Geometry check sheet. Reference: drawing and pictorial views, mm from the part's lowest x, y, z. A direction names the side the tool comes from. Round coordinates to 2 decimals unless told otherwise and drop trailing zeros. Write each loop counter-clockwise with the first axis right and the second up, starting at its lowest first coordinate (ties: lowest second). Pieces come first, ordered by that corner, then holes. Notation, with made-up numbers: (67.5, 11) - (101.5, 11) arc R21 ccw to (101.5, 38) - close; hole circle Ø10 at (6.25, -18.75). An arc over 180 degrees is marked (long way). Return JSON: item names as keys, results as strings.
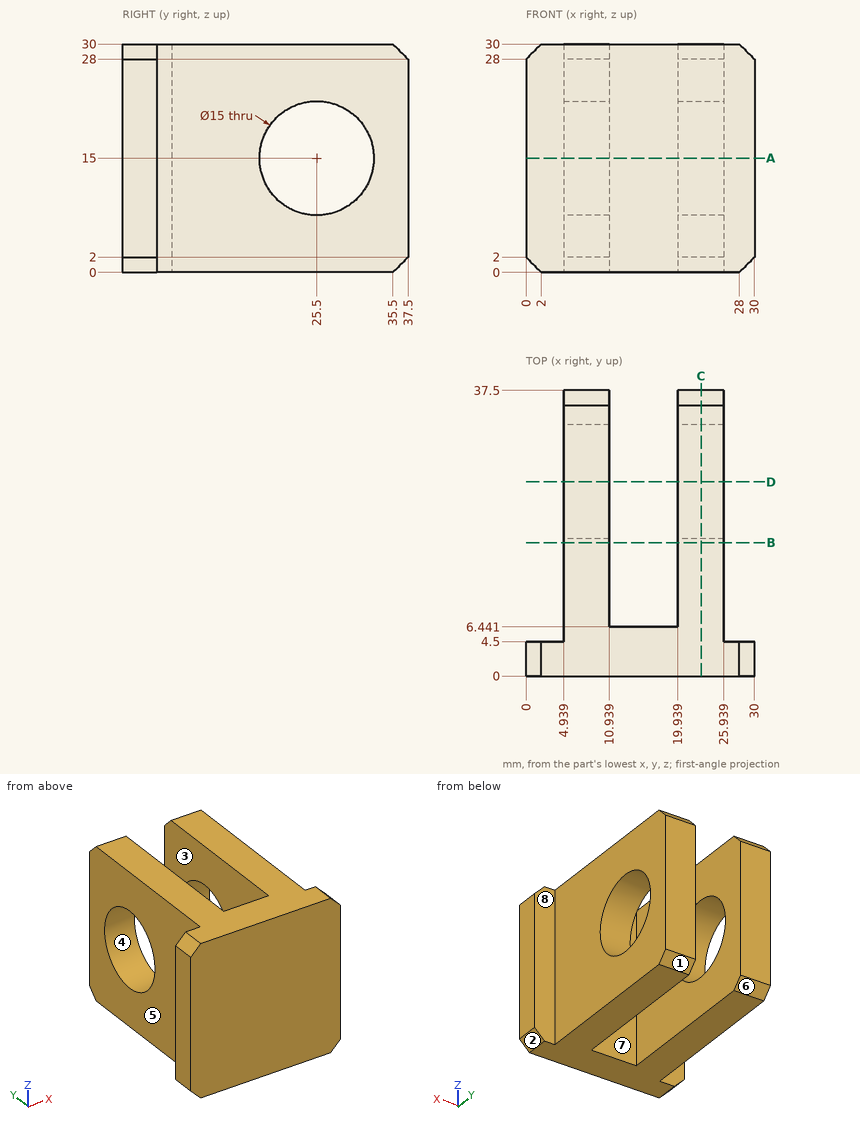
(1) Access from +Z, -Z, +X, -X, +Y, -Y to the whole of each face (thin tool, end or side, straight path). Record for the marked faces 4, 5, 6, 7 and 8.
Response values:
{"face 4": "+X, -X", "face 5": "+Z, -Z, -X, +Y", "face 6": "-Z, +X, -X, +Y", "face 7": "+Z, -Z, +Y", "face 8": "+Z, -Z, +X, +Y"}
(2) Section check D-D, the plane y = 25.5. Enter the section's corners in (x, z).
Response values:
{"outline": "(4.94, 0) - (10.94, 0) - (10.94, 7.5) - (4.94, 7.5) - close; (4.94, 22.5) - (10.94, 22.5) - (10.94, 30) - (4.94, 30) - close; (19.94, 0) - (25.94, 0) - (25.94, 7.5) - (19.94, 7.5) - close; (19.94, 22.5) - (25.94, 22.5) - (25.94, 30) - (19.94, 30) - close"}
(3) Section check A-A, the plane z = 15. Enter the section's corners in (x, y).
Response values:
{"outline": "(0, 0) - (30, 0) - (30, 4.5) - (25.94, 4.5) - (25.94, 18) - (19.94, 18) - (19.94, 6.44) - (10.94, 6.44) - (10.94, 18) - (4.94, 18) - (4.94, 4.5) - (0, 4.5) - close; (4.94, 33) - (10.94, 33) - (10.94, 37.5) - (4.94, 37.5) - close; (19.94, 33) - (25.94, 33) - (25.94, 37.5) - (19.94, 37.5) - close"}
(4) Gauge pin test, flat ends, axial feed: pin 1 (15 mm diameter, centred on y = 19.5, z = 19, fed in from +X); pin 2 (4.5 mm diameter, centred on x = 29, z = 15, fed in from +Y); pin 3 (7 mm diameter, centred on x = 16, z = 22.5, fed in from +Y). Record the tip position at first contact, or that the pin passes through.
Response values:
{"pin 1": "stops at x = 25.94", "pin 2": "stops at y = 4.5", "pin 3": "stops at y = 6.44"}
(5) Release check for a two-part mould opening along X. For the marked faces 1, 2 and 3 record: pulls with the +X half, pulls with the -X half, needs draft (parallel to the pull), parting line crosses it, or undercut.
Response values:
{"face 1": "needs draft", "face 2": "pulls with the +X half", "face 3": "undercut"}
(6) Section check C-C, the plane x = 23. Enter the section's corners in (y, z), plus the area to 3 significant figures.
Response values:
{"outline": "(0, 0) - (35.5, 0) - (37.5, 2) - (37.5, 28) - (35.5, 30) - (0, 30) - close; hole circle Ø15 at (25.5, 15)", "area": "944 mm^2"}
(7) Material ranges on line 1 along Y through (x, z) = (9.5, 15); line 2 along X through (y, z) = (24, 28.5); line 3 along Y through (x, z) = (28, 11.5), recorded low to high. Write a range as [from, to].
Response values:
{"line 1": "y = [0, 18], [33, 37.5]", "line 2": "x = [4.94, 10.94], [19.94, 25.94]", "line 3": "y = [0, 4.5]"}
(8) Section check B-B, the plane y = 17.5. Enter the section's corners in (x, z), plus the area to 3 significant figures.
Response values:
{"outline": "(4.94, 0) - (10.94, 0) - (10.94, 30) - (4.94, 30) - close; (19.94, 0) - (25.94, 0) - (25.94, 30) - (19.94, 30) - close", "area": "360 mm^2"}
